Geometry: see drawing. Coordinates: mm, zero at the bounding-box minimum. Give positions to 0.01 mm unless a question says otherwise; leave off trailing zeros. Loops run counter-clockwise (first coordinate to the right, second up) from the corner with the lowest first, then second, coordinate; pieces in that order, holes last. Notation, with made-up numbers: (43.5, 67) -> (61.5, 67) arc R7 ccw to (61.5, 76) -> close; hole circle Ø2 at (65.25, 20). An arc over 180 degrees is marked (long way). Answer in a Markdown table with one row per item. Add a question column.
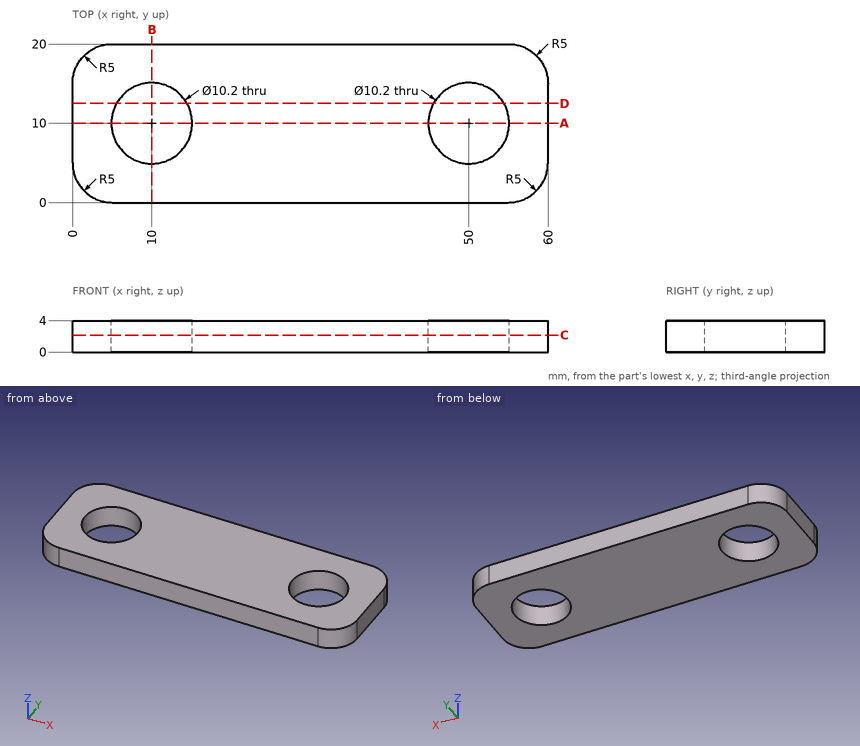
1) Material intervals for line 1 along X through (y, z) = (12.5, 2.4); line 2 along Y through (x, z) = (50, 2.4); line 3 along X through (y, z) = (13, 1), sorted ascending.
2) Section A-A on y = 10. Output: boundary loops of the cut face in (x, z).
3) Pin query (flat end, axial travel): pin 1 (8 mm diameter, centred on x = 50, y = 10, fed in from -Z). Return the tip coordinate at first contact, or that it passes through.
4) Section D-D on y = 12.5. Output: boundary loops of the cut face in (x, z).
5) Section B-B on x = 10. Output: boundary loops of the cut face in (y, z), and give its area (3 significant figures).
6) Section C-C on z = 2.15. Output: boundary loops of the cut face in (x, y).
Working result:
| question | item | result |
|---|---|---|
| 1 | line 1 | x = 0 to 5.55, 14.45 to 45.55, 54.45 to 60 |
| 1 | line 2 | y = 0 to 4.9, 15.1 to 20 |
| 1 | line 3 | x = 0 to 5.88, 14.12 to 45.88, 54.12 to 60 |
| 2 | outline | (0, 0) -> (4.9, 0) -> (4.9, 4) -> (0, 4) -> close; (15.1, 0) -> (44.9, 0) -> (44.9, 4) -> (15.1, 4) -> close; (55.1, 0) -> (60, 0) -> (60, 4) -> (55.1, 4) -> close |
| 3 | pin 1 | passes through |
| 4 | outline | (0, 0) -> (5.55, 0) -> (5.55, 4) -> (0, 4) -> close; (14.45, 0) -> (45.55, 0) -> (45.55, 4) -> (14.45, 4) -> close; (54.45, 0) -> (60, 0) -> (60, 4) -> (54.45, 4) -> close |
| 5 | outline | (0, 0) -> (4.9, 0) -> (4.9, 4) -> (0, 4) -> close; (15.1, 0) -> (20, 0) -> (20, 4) -> (15.1, 4) -> close |
| 5 | area | 39.2 mm2 |
| 6 | outline | (0, 5) arc R5 ccw to (5, 0) -> (55, 0) arc R5 ccw to (60, 5) -> (60, 15) arc R5 ccw to (55, 20) -> (5, 20) arc R5 ccw to (0, 15) -> close; hole circle Ø10.2 at (10, 10); hole circle Ø10.2 at (50, 10) |
